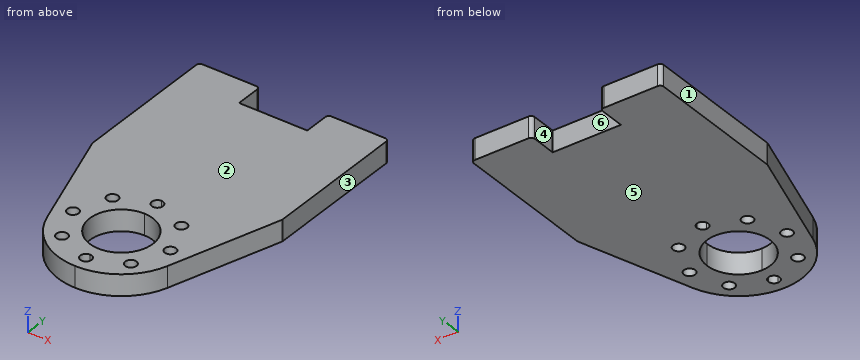
from build123d import *

# Parameters (mm, degrees)
ESQUISSE1_R        = 0.8
BOSS_EXTRU_1_DEPTH = 3
CONG_1_R           = 0.5


with BuildPart() as part:
    # Esquisse1 → Boss.-Extru.1 (new body)
    # profile 1 of 4: a face of its own
    with BuildSketch(Plane.XY):
        with BuildLine():
            Line((-13.5, 4), (-13.5, 0))
            Line((-13.5, 0), (-13.5, -16.644680961))
            Line((-13.5, -16.644680961), (-8.580913976, -32.195227318))
            ThreePointArc((-8.580913976, -32.195227318), (-7.260492881, -24.162449633), (0, -20.4808369))
            Line((0, -20.4808369), (0, 0))
            Line((0, 0), (-4.85, 0))
            Line((-4.85, 0), (-4.85, 4))
            Line((-4.85, 4), (-13.5, 4))
        make_face()
    # profile 2 of 4: a face of its own
    with BuildSketch(Plane.XY):
        with BuildLine():
            Line((0, 0), (0, -20.4808369))
            ThreePointArc((0, -20.4808369), (6.363961031, -23.11687587), (9, -29.4808369))
            ThreePointArc((9, -29.4808369), (8.894611453, -30.85411295), (8.580913976, -32.195227318))
            Line((8.580913976, -32.195227318), (13.5, -16.644680961))
            Line((13.5, -16.644680961), (13.5, 0))
            Line((13.5, 0), (13.5, 4))
            Line((13.5, 4), (4.85, 4))
            Line((4.85, 4), (4.85, 0))
            Line((4.85, 0), (0, 0))
        make_face()
    # profile 3 of 4: a face of its own
    with BuildSketch(Plane.XY):
        with BuildLine():
            ThreePointArc((9, -29.4808369), (6.363961031, -23.11687587), (0, -20.4808369))
            Line((0, -20.4808369), (0, -21.6808369))
            ThreePointArc((0, -21.6808369), (0.565685425, -21.915151475), (0.8, -22.4808369))
            ThreePointArc((0.8, -22.4808369), (0.565685425, -23.046522325), (0, -23.2808369))
            Line((0, -23.2808369), (0, -24.9808369))
            ThreePointArc((0, -24.9808369), (3.181980515, -26.298856385), (4.5, -29.4808369))
            ThreePointArc((4.5, -29.4808369), (3.181980515, -32.662817416), (0, -33.9808369))
            Line((0, -33.9808369), (0, -35.539601481))
            ThreePointArc((0, -35.539601481), (0.565685425, -35.773916056), (0.8, -36.339601481))
            ThreePointArc((0.8, -36.339601481), (0.565685425, -36.905286906), (0, -37.139601481))
            Line((0, -37.139601481), (0, -38.4808369))
            ThreePointArc((0, -38.4808369), (5.318387267, -36.741329781), (8.580913976, -32.195227318))
            ThreePointArc((8.580913976, -32.195227318), (8.894611453, -30.85411295), (9, -29.4808369))
        make_face()
        with Locations((4.899813207, -34.310032397)):
            Circle(ESQUISSE1_R, mode=Mode.SUBTRACT)
        with Locations((6.92938229, -29.410219191)):
            Circle(ESQUISSE1_R, mode=Mode.SUBTRACT)
        with Locations((4.899813207, -24.510405984)):
            Circle(ESQUISSE1_R, mode=Mode.SUBTRACT)
    # profile 4 of 4: a face of its own
    with BuildSketch(Plane.XY):
        with BuildLine():
            ThreePointArc((0, -20.4808369), (-7.260492881, -24.162449633), (-8.580913976, -32.195227318))
            ThreePointArc((-8.580913976, -32.195227318), (-5.318387267, -36.741329781), (0, -38.4808369))
            Line((0, -38.4808369), (0, -37.139601481))
            ThreePointArc((0, -37.139601481), (-0.8, -36.339601481), (0, -35.539601481))
            Line((0, -35.539601481), (0, -33.9808369))
            ThreePointArc((0, -33.9808369), (-4.5, -29.4808369), (0, -24.9808369))
            Line((0, -24.9808369), (0, -23.2808369))
            ThreePointArc((0, -23.2808369), (-0.8, -22.4808369), (0, -21.6808369))
            Line((0, -21.6808369), (0, -20.4808369))
        make_face()
        with Locations((-6.92938229, -29.410219191)):
            Circle(ESQUISSE1_R, mode=Mode.SUBTRACT)
        with Locations((-4.899813207, -34.310032397)):
            Circle(ESQUISSE1_R, mode=Mode.SUBTRACT)
        with Locations((-4.899813207, -24.510405984)):
            Circle(ESQUISSE1_R, mode=Mode.SUBTRACT)
    extrude(amount=BOSS_EXTRU_1_DEPTH)

    # Congé1
    cong_1_edges = [part.edges().sort_by_distance(p)[0] for p in [
        (-13.5, -16.644680961, 1.5),
        (-13.5, 4, 1.5),
        (-4.85, 4, 1.5),
        (4.85, 4, 1.5),
        (13.5, 4, 1.5),
        (13.5, -16.644680961, 1.5),
    ]]
    fillet(cong_1_edges, radius=CONG_1_R)


solid = part.part
Check sheet for the modelled part. Datum: model origin and axes. Units: mm. Face numbers are marked on the shaded views. A direction names the side the tool comes from. Round coordinates to 2 decimals unless told otherwise and drop trailing zeros. Write each loop counter-clockwise with the first axis right and the second up, starting at its lowest first coordinate (ties: lowest second). Pieces come first, ordered by that corner, then holes. Notation, with made-up numbers: (-9, 9) - (33, 9) arc R26 ccw to (33, 35) - close; hole circle Ø1 at (17.5, 16). An arc over 180 degrees is marked (long way). Return JSON: item names as keys, results as strings.
Q1. Depth check by flat-ended pin: P1, Ø1.4, axis at x = 4.9, y = -34.31, coming from the +Z side. Enter the tip coordinate at first touch or a pass-through.
Returned:
{"P1": "passes through"}
Q2. Scan lines: L1, parallel to X at y = 2, z = 0.9; L2, parallel to Y at x = -5.5, z = 2.35; L3, parallel to Y at x = 7, z = 1.35. Record each from-to range of solid material in increasing order. Write a range as from..to.
Returned:
{"L1": "x = -13.5..-4.85, 4.85..13.5", "L2": "y = -36.6..-34.84, -33.78..-25.04, -23.98..4", "L3": "y = -35.14..-30.21, -28.61..4"}
Q3. Cross-section at B-B (z = 1.5). Give the number of separate pieces and of enclosed holes in the cut face, then the cut area to 3 significant figures.
Returned:
{"separate pieces": "1", "enclosed holes": "9", "area": "861 mm²"}
Q4. Cross-section at A-A (x = -3). Record the boundary of the cut face in (y, z), then the cut area to 3 significant figures.
Returned:
{"outline": "(-37.97, 0) - (-32.83, 0) - (-32.83, 3) - (-37.97, 3) - close; (-26.13, 0) - (0, 0) - (0, 3) - (-26.13, 3) - close", "area": "93.8 mm²"}
Q5. Access from +Z, -Z, +X, -X, +Y, -Y to the whole of each face (thin tool, end or side, straight path). Record for the marked faces 5 and 6.
Returned:
{"face 5": "-Z, +X, -X, +Y, -Y", "face 6": "+Z, -Z, +Y"}
Q6. Draft check along X on the marked faces 1, 2, 3 and 4. Enter one of: released by +X, released by -X, zero draft, split by the parting line, or undercut.
Returned:
{"face 1": "released by -X", "face 2": "zero draft", "face 3": "released by +X", "face 4": "undercut"}
Q7. Cross-section at D-D (x = 10.75). Record the boundary of the cut face in (y, z), then the cut area to 3 significant figures.
Returned:
{"outline": "(-25.34, 0) - (4, 0) - (4, 3) - (-25.34, 3) - close", "area": "88.0 mm²"}
Q8. Cross-section at C-C (x = 2.5). Record the boundary of the cut face in (y, z).
Returned:
{"outline": "(-38.13, 0) - (-33.22, 0) - (-33.22, 3) - (-38.13, 3) - close; (-25.74, 0) - (0, 0) - (0, 3) - (-25.74, 3) - close"}
